Part print with two shaded views. Sizes in mm from the minimum x, y, z corner. A direction names the side the tool comes from. Round coordinates to 2 decimals unless told otherwise and drop trailing zeros. Loops run counter-clockwise (first coordinate to the right, second up) from the corner with the lowest first, then second, coordinate; pieces in that order, holes last. Notation, with made-up numbers: M 13,-35 L 44,-35 A21 ccw 44,-13 Z; hole C 85,-10.5 d1. An arc over 180 degrees is marked long. Answer as CSV lines item,"result". Start each with the question number.
Item 1: Band-saw the part on A-A (x = 50.8). Give the cut face in (y, z) (3 decimals), and give its area (3 significant figures).
Item 2: Wall check: line 1 (X direction, y = 22.5, z = 6.35) (3 decimals); line 2 (Z direction, x = 44.45, y = 23.75) (3 decimals); line 3 (X direction, y = 19.5, z = 8). Give the ranges that are in metal, low to high.
Item 3: Which spindle directions (+Z, -Z, +X, -X, +Y, -Y) get a long thin tool onto all of the face, cutting with end or side? Do the marked faces 4, 5 and 6. Say none if no direction does.
Item 4: Mould opens along Z. For the marked faces 1, 2 and 3 say: pulls with the +Z half, pulls with the -Z half, needs draft (parallel to the pull), parting line crosses it, or undercut.
Item 5: Band-saw the part on B-B (z = 6.35). Give the cut face in (x, y) (3 decimals).
Item 6: Band-saw the part on C-C (y = 20). Give the cut face in (x, z) (3 decimals).
Item 7: Drop a flat-ended pin along its axis: pin 1 Ø3 at (x, z) = (32.5, 7) entering from +Y. Give the stop position or say it passes through.
Item 8: Band-saw the part on D-D (y = 4.75). Give the cut face in (x, z) (3 decimals).
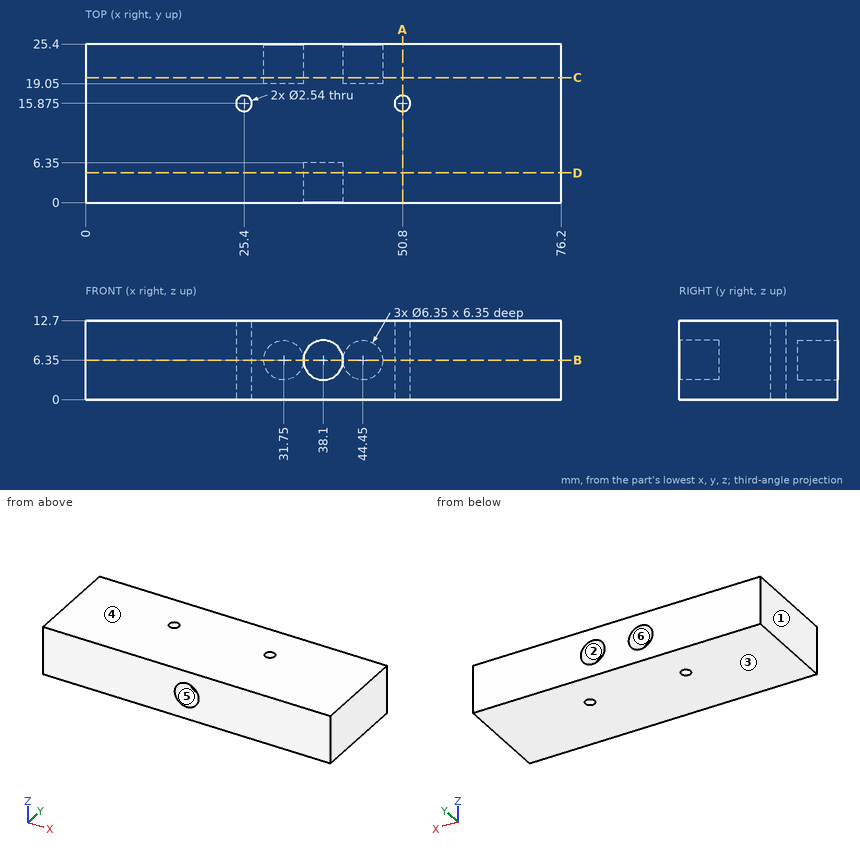
Answer block:
1,outline,"M 0,0 L 14.605,0 L 14.605,12.7 L 0,12.7 Z; M 17.145,0 L 25.4,0 L 25.4,12.7 L 17.145,12.7 Z"
1,area,"290 mm^2"
2,line 1,"x = 0 to 28.575, 34.925 to 41.275, 47.625 to 76.2"
2,line 2,"z = 0 to 3.175, 9.525 to 12.7"
2,line 3,"x = 0 to 29.04, 34.46 to 41.74, 47.16 to 76.2"
3,face 4,"+Z, +X, -X, +Y, -Y"
3,face 5,"-Y"
3,face 6,"+Y"
4,face 1,"needs draft"
4,face 2,"undercut"
4,face 3,"pulls with the -Z half"
5,outline,"M 0,0 L 34.925,0 L 34.925,6.35 L 41.275,6.35 L 41.275,0 L 76.2,0 L 76.2,25.4 L 47.625,25.4 L 47.625,19.05 L 41.275,19.05 L 41.275,25.4 L 34.925,25.4 L 34.925,19.05 L 28.575,19.05 L 28.575,25.4 L 0,25.4 Z; hole C 25.4,15.875 d2.54; hole C 50.8,15.875 d2.54"
6,outline,"M 0,0 L 76.2,0 L 76.2,12.7 L 0,12.7 Z; hole C 31.75,6.35 d6.35; hole C 44.45,6.35 d6.35"
7,pin 1,"stops at y = 19.05"
8,outline,"M 0,0 L 76.2,0 L 76.2,12.7 L 0,12.7 Z; hole C 38.1,6.35 d6.35"
